Build history of the part. All positions in model axes, mm. A direction names the side the tool comes from. Round coordinates to 2 decimals unless told otherwise and drop trailing zeros. Write each loop counter-clockwise with the first axis right and the second up, starting at its lowest first coordinate (ties: lowest second). Pieces come first, ordered by that corner, then holes. Notation, with made-up numbers: (66.5, -16) - (71.5, -16) arc R25 cw to (71.5, 1) - close; hole circle Ø1 at (-1.75, 55). An arc over 180 degrees is marked (long way). Answer as a JSON object with one key per item and string values. Group by question number.
Item 1: Slice it at C-C, the plane z = 1.3. List the corners of the cut face in (x, y).
Item 2: Probe line 1 (X direction, y = 11.25, z = 3.1); line 2 (Z direction, x = 8.5, y = -8.5); line 3 (Y direction, x = 7, z = 2.1). List the from-to ranges inside material, lowest first. Write a range as from..to.
Item 3: Slice it at A-A, the plane y = 0. List the corners of the cut face in (x, z), then the cut area to 3 significant figures.
Item 4: Two-plate mould, pull along X, no slides. Class faces 1 (the cylindrical face through (12.08, -6.55, 2.99)), 2 (the cylindrical face through (-12.48, 8.32, 2.99)), 3 (the cylindrical face through (0, -2.6, 2)): +X half, -X half, draft (parallel to the pull), parting line (faces both ways), or undercut.
Item 5: Which spindle directions (+Z, -Z, +X, -X, +Y, -Y) get a long thin tool onto all of the face, cutting with end or side? Do faces 4 (the cylindrical face through (12.11, 6.58, 2.99)), 5 (the flat face through (1.6, 0, 2)), 6 (the cylindrical face through (-6.58, 12.11, 2.99)), 7 (the cylindrical face through (-12.08, 6.55, 2.99)). Say none if no direction does.
Item 6: Slice it at D-D, the plane y = 4.5. List the corners of the cut face in (x, z), then the cut area to 3 significant figures.
Item 7: Flat gauge pins, fed straight in: pin 1 (1 mm diameter, centred on x = 10, z = 3, fed in from -Y); pin 2 (2 mm diameter, centred on y = -0.5, z = 3, fed in from -X). Where does each tip first touch, or does it go through?
Item 8: Slice it at B-B, the plane x = 0. List the corners of the cut face in (y, z).
Autodesk Inventor part; units mm, degrees
ref_plane "YZ Plane" through (0, 0, 0) normal (1, 0, 0) x (0, 1, 0)
ref_plane "XY Plane" through (0, 0, 0) normal (0, 0, 1) x (1, 0, 0)
sketch "Skizze1" plane through (0, 0, 0) normal (0, 0, 1) x (1, 0, 0)
  circle A0 centre (0, 0) radius 2.6
  circle A1 centre (0, 0) radius 15
  line L0 (-1.6, 2.0494) -> (-1.6, -2.0494)
  line L1 (1.6, -2.0494) -> (1.6, 2.0494)
  dimension "d0" = 5.2
  dimension "d1" = 30
  dimension "d2" = 3.2
extrude "Extrusion1" add sketch "Skizze1" along normal blind 4 contours A0 L1 | L0 A0 | A1
sketch "Skizze3" plane through (0, 0, 0) normal (0, 0, -1) x (-1, 0, 0)
  circle A0 centre (0, 0) radius 5
  circle A1 centre (0, 0) radius 15
  dimension "d8" = 10
  dimension "d9" = 30
extrude "Extrusion3" cut sketch "Skizze3" against normal blind 2
sketch "Skizze4" plane through (0, 0, 2) normal (0, 0, -1) x (-1, 0, 0)
  circle A0 centre (0, 0) radius 12.5 construction
  circle A1 centre (0, 0) radius 15
  line L0 (-15, 0) -> (-12.5, 0)
  arc A2 (-12.4599, -1) -> (-14.8661, -2) centre (-8.8919, -12.9799) ccw
  arc A3 (-14.8661, 2) -> (-12.4599, 1) centre (-8.8919, 12.9799) ccw
  arc A4 (-14.8661, 2) -> (-14.8661, -2) centre (0, 0) ccw
  arc A5 (-12.4599, 1) -> (-12.4599, -1) centre (0, 0) ccw
  circle A6 centre (0, 0) radius 15
  point P0 (-13.75, 0)
  dimension "d12" = 25
  dimension "d13" = 12.5
  dimension "d14" = 4
  dimension "d15" = 2
extrude "Extrusion4" cut sketch "Skizze4" against normal blind 2 contours A3 A5 L0 A1 | A1 L0 A5 A2
pattern_circular "Runde Anordnung1" count 16 over 360 about axis through (0, 0, 0) along (0, 0, 1) of "Extrusion4"
ref_plane "Arbeitsebene1" through (0, 16.5, 0) normal (0, 1, 0) x (-1, 0, 0)
properties part number "Adapter Stepper"
Geometry says:
{
 "1": {"outline": "circle Ø10 at (0, 0); hole (-1.6, -2.05) arc R2.6 ccw to (1.6, -2.05) - (1.6, 2.05) arc R2.6 ccw to (-1.6, 2.05) - close"},
 "2": {"line 1": "x = -8.88..-5.79, -5.45..5.45, 5.79..8.88", "line 2": "z = 2..4", "line 3": "y = -12.51..12.51"},
 "3": {"outline": "(-12.5, 2) - (-5, 2) - (-5, 0) - (-1.6, 0) - (-1.6, 4) - (-12.5, 4) - close; (1.6, 0) - (5, 0) - (5, 2) - (12.5, 2) - (12.5, 4) - (1.6, 4) - close", "area": "57.2 mm^2"},
 "4": {"face 1": "+X half", "face 2": "-X half", "face 3": "undercut"},
 "5": {"face 4": "+Z, -Z, +X", "face 5": "+Z, -Z", "face 6": "+Z, -Z, +Y", "face 7": "+Z, -Z, -X"},
 "6": {"outline": "(-11.66, 2) - (-2.18, 2) - (-2.18, 0) - (2.18, 0) - (2.18, 2) - (11.66, 2) - (11.66, 4) - (-11.66, 4) - close", "area": "55.4 mm^2"},
 "7": {"pin 1": "stops at y = -8.58", "pin 2": "stops at x = -13.84"},
 "8": {"outline": "(-12.5, 2) - (-5, 2) - (-5, 0) - (-2.6, 0) - (-2.6, 4) - (-12.5, 4) - close; (2.6, 0) - (5, 0) - (5, 2) - (12.5, 2) - (12.5, 4) - (2.6, 4) - close"}
}
